The listing builds one solid part. Answer for the finished solid, in the listing's coordinates (mm). A direction names the side the tool comes from. Coordinates: 2 decimals unless noted, no trailing zeros. Write each loop counter-clockwise with the first axis right and the second up, starting at its lowest first coordinate (ties: lowest second). Pieces come first, ordered by that corner, then holes. Notation, with made-up numbers: M 29.25,9.25 L 43.25,9.25 A26 ccw 43.25,28.25 Z; hole C 37.5,65 d5. An arc over 180 degrees is marked long. Answer as CSV lines item,"result".
Autodesk Inventor part; units mm, degrees
ref_plane "YZ Plane" through (0, 0, 0) normal (1, 0, 0) x (0, 1, 0)
ref_plane "XZ Plane" through (0, 0, 0) normal (0, 1, 0) x (-1, 0, 0)
ref_plane "XY Plane" through (0, 0, 0) normal (0, 0, 1) x (1, 0, 0)
sketch "스케치1" plane through (0, 0, 0) normal (0, 0, 1) x (1, 0, 0)
  circle A0 centre (0, 0) radius 2.725
  dimension "d0" = 5.45
extrude "돌출1" add sketch "스케치1" along normal blind 13.8
sketch "스케치2" plane through (0, 0, 13.8) normal (0, 0, 1) x (1, 0, 0)
  circle A0 centre (0, 0) radius 1.075
  dimension "d3" = 2.15
extrude "돌출2" cut sketch "스케치2" against normal blind 20.45
fillet "모깎기1" radius 1 1 edges at (-2.725, 0, 13.8)
sketch "스케치3" plane through (0, 0, 0) normal (0, 0, -1) x (-1, 0, 0)
  circle A0 centre (0, 0) radius 4.475
  dimension "d7" = 8.95
extrude "돌출3" add sketch "스케치3" along normal blind 22.7
sketch "스케치4" plane through (0, 0, -22.7) normal (0, 0, -1) x (-1, 0, 0)
  circle A0 centre (0, 0) radius 1.075
  circle A1 centre (0, 0) radius 3
  dimension "d10" = 6
extrude "돌출4" cut sketch "스케치4" against normal blind 18.8 contours A0 | A1
properties part number "DC_PLUG"
Q1. For faces 5 (the flat face through (-1, -3, -22.7)), 6 (the cylindrical face through (3, 0, -13)), 7 (the flat face through (0, -3, 0)), determine the directions among +Z, -Z, +X, -X, +Y, -Y from which every point of the face is accessible in a straight line to the end or side of a thin tool.
Output:
face 5,"-Z, +X, -X, +Y, -Y"
face 6,"-Z"
face 7,"+Z"
Q2. The mould has two halves that part along Y. Classify faces 1 (the cylindrical face through (3.551, 2.723, -11.191)), 2 (the flat face through (1, 1, 13.8)), 3 (the cylindrical face through (-1.074, 0.047, 6.997)), 4 (the flat face through (0, 0, 0)): pulls with the +Y half, pulls with the -Y half, needs draft (parallel to the pull), parting line crosses it, or undercut.
Output:
face 1,"parting line crosses it"
face 2,"needs draft"
face 3,"undercut"
face 4,"undercut"
Q3. Flat-ended cylindrical pins translate along their axes: pin 1 Ø2 at (y, z) = (-3, -8) entering from -X; pin 2 Ø1.9 at (x, y) = (0, 0) entering from +Z; pin 3 Ø3 at (x, y) = (-0.5, 0.5) entering from -Z; pin 4 Ø3 at (x, y) = (-2, -2.5) entering from +Z. Find the tip coordinate at first contact, or state that the pin passes through.
Output:
pin 1,"x = -4"
pin 2,"z = 0"
pin 3,"z = -3.9"
pin 4,"z = 13.8"
Q4. Straight lines are drawn through the part: line 1 (Y direction, x = 0, z = -10) (3 decimals); line 2 (Y direction, x = 0, z = 4) (3 decimals); line 3 (Z direction, x = 1.5, y = -3.25). For each, find the intervals that lie inside material, in ascending order.
Output:
line 1,"-4.475 to -3, 3 to 4.475"
line 2,"-2.725 to -1.075, 1.075 to 2.725"
line 3,"-22.7 to 0"
Q5. Find section C-C (z = 10.5). Give the vertices of the cut face in (x, y) (3 decimals).
Output:
outline,"C 0,0 d5.45; hole C 0,0 d2.15"
Q6. Find section D-D (x = -3.5). Give the vertices of the cut face in (y, z), and give its area (3 significant figures).
Output:
outline,"M -2.79,-22.7 L 2.79,-22.7 L 2.79,0 L -2.79,0 Z"
area,"127 mm2"
Q7. Find section A-A (y = 0). Give the vertices of the cut face in (x, z) (3 decimals).
Output:
outline,"M -4.475,-22.7 L -3,-22.7 L -3,-3.9 L 3,-3.9 L 3,-22.7 L 4.475,-22.7 L 4.475,0 L 2.725,0 L 2.725,12.8 A1 ccw 1.725,13.8 L 1.075,13.8 L 1.075,0 L -1.075,0 L -1.075,13.8 L -1.725,13.8 A1 ccw -2.725,12.8 L -2.725,0 L -4.475,0 Z"
